Verification items for the finished model (mm, model axes). A direction names the side the tool comes from. Coordinates: 2 decimals unless noted, no trailing zeros. Order: outer loops, then holes, each group sorted by start corner. A loop starts at its lowest first (then second) coordinate and runs counter-clockwise, first axis right, second up. Notation, with made-up numbers: (47, 78.25) -> (72, 78.25) arc R9 cw to (72, 82.25) -> close; hole circle Ø10 at (40, 10). An arc over 180 degrees is marked (long way). Write item = value, one per line. Start each with the question number.
1. Release check for a two-part mould opening along Y. For faces 4 (the cylindrical face through (-2.217, -2.199, 3.369)), 5 (the cylindrical face through (51.406, -1.926, 3.607)), 6 (the flat face through (27, -2, 4.233)), 7 (the flat face through (26, -4.233, 2)) record: +Y half, -Y half, draft (parallel to the pull), parting line (faces both ways), or undercut.
2. Go/stop test with flat-tipped pins: P1, Ø1.3, axis at x = -1, z = 1, coming from the +Y side; P2, Ø1.3, axis at x = 26.5, y = -2.5, coming from the +Z side; P3, Ø1, axis at x = 50.8, y = -2.12, coming from the -Z side. Record where each tip stops, or that it passes through.
3. Cross-section at A-A on z = 0.6. Record the cut outline in (x, y) (1 decimal).
4. Cross-section at B-B on x = 16.5. Record the cut outline in (y, z), plus the area to 3 significant figures.
5. Thickness scan on line 1 along X through (y, z) = (-2.2, 2.35); line 2 along Z through (x, y) = (26, -1.6); line 3 along X through (y, z) = (-2, 0.7). Record the ranges inside material, lowest first. Write a range as from..to.
6. Set-up check for faces 1 (the flat face through (-1, -0.529, 1)), 2 (the flat face through (-0.86, -1.79, 2.117)), 3 (the flat face through (-1, -3.704, 1)): record each of +Z, -Z, +X, -X, +Y, -Y from which the full face is reachable in a straight line by a thin tool's end or side.
from build123d import *

# Parameters (mm, degrees)
BOSS_EXTRUDE3_DEPTH = 4.233333333
SKETCH4_W           = 2.116666667
SKETCH4_H           = 3.175
BOSS_EXTRUDE5_DEPTH = 3.175
CUT_EXTRUDE1_START  = -2.116666667
CUT_EXTRUDE1_DEPTH  = 2.116666667
SKETCH6_R           = 0.635
BOSS_EXTRUDE6_DEPTH = 2.54
SKETCH7_R           = 0.635
CUT_EXTRUDE2_DEPTH  = 1.27
CUT_EXTRUDE3_START  = -1.27
SKETCH8_R           = 0.635
CUT_EXTRUDE3_DEPTH  = 1.27


# Read off the part's stored shape, not the designer's step: Cut-Extrude1
with BuildPart() as part:
    # Sketch3 → Boss-Extrude3 (new body)
    with BuildSketch(Plane.XY):
        with BuildLine():
            Line((0, 0), (50.8, 0))
            ThreePointArc((50.8, 0), (52.916666667, -2.116666667), (50.8, -4.233333333))
            Line((50.8, -4.233333333), (0, -4.233333333))
            Line((0, -4.233333333), (0, 0))
        make_face()
    extrude(amount=BOSS_EXTRUDE3_DEPTH)

    # Sketch4 → Boss-Extrude5 (add)
    with BuildSketch(Plane.ZY):
        with Locations((1.058333334, -2.116666667)):
            Rectangle(SKETCH4_W, SKETCH4_H)
    extrude(amount=BOSS_EXTRUDE5_DEPTH)

    # Cut-Extrude1 outline → Cut-Extrude1 (cut)
    with BuildSketch(Plane(origin=(0, 0, 0), x_dir=(-1, 0, 0), z_dir=(0, 0, -1)).offset(CUT_EXTRUDE1_START)):
        with BuildLine():
            Line((3.175, -0.529166667), (1.5875, -0.529166667))
            ThreePointArc((1.5875, -0.529166667), (2.710032015, -0.994134652), (3.175, -2.116666667))
            Line((3.175, -2.116666667), (3.175, -0.529166667))
        make_face()
        with BuildLine():
            Line((3.175, -3.704166667), (3.175, -2.116666667))
            ThreePointArc((3.175, -2.116666667), (2.710032015, -3.239198682), (1.5875, -3.704166667))
            Line((1.5875, -3.704166667), (3.175, -3.704166667))
        make_face()
    extrude(amount=CUT_EXTRUDE1_DEPTH, mode=Mode.SUBTRACT)

    # Sketch6 → Boss-Extrude6 (add)
    with BuildSketch(Plane.XY.offset(2.116666667)):
        with Locations(Location((-1.5875, -2.116666667, 0), (0, 0, 90))):
            Circle(SKETCH6_R)
    extrude(amount=BOSS_EXTRUDE6_DEPTH)

    # Sketch7 → Cut-Extrude2 (cut)
    with BuildSketch(Plane.XY.offset(4.233333333)):
        with Locations((50.8, -2.116666667)):
            Circle(SKETCH7_R)
    extrude(amount=-CUT_EXTRUDE2_DEPTH, mode=Mode.SUBTRACT)

    # Sketch8 → Cut-Extrude3 (cut)
    with BuildSketch(Plane(origin=(0, 0, 0), x_dir=(-1, 0, 0), z_dir=(0, 0, -1)).offset(CUT_EXTRUDE3_START)):
        with Locations(Location((-50.8, -2.116666667, 0), (0, 0, 180))):
            Circle(SKETCH8_R)
    extrude(amount=CUT_EXTRUDE3_DEPTH, mode=Mode.SUBTRACT)


solid = part.part
Worked out:
q1.face_4 = parting line
q1.face_5 = undercut
q1.face_6 = draft
q1.face_7 = -Y half
q2.P1 = -0.53
q2.P2 = 4.23
q2.P3 = 1.27
q3.outline = (-1.6, -3.7) -> (0, -3.7) -> (0, -4.2) -> (50.8, -4.2) arc R2.1 ccw to (50.8, 0) -> (0, 0) -> (0, -0.5) -> (-1.6, -0.5) arc R1.6 ccw to start; hole circle Ø1.3 at (50.8, -2.1)
q4.outline = (-4.23, 0) -> (0, 0) -> (0, 4.23) -> (-4.23, 4.23) -> close
q4.area = 17.9 mm²
q5.line_1 = -2.22..-0.96, 0..52.92
q5.line_2 = 0..4.23
q5.line_3 = -3.17..50.18, 51.42..52.91
q6.face_1 = +Z, -Z, -X, +Y
q6.face_2 = +Z
q6.face_3 = +Z, -Z, -X, -Y
